from build123d import *

# Parameters (mm, degrees)
SKETCH_1_W            = 65
SKETCH_1_H            = 72
EXTRUDE_1_DEPTH       = 50
SKETCH_2_W            = 28
SKETCH_2_H            = 50
CUT_EXTRUDE_1_DEPTH   = 94.489304201
SKETCH_4_W            = 65
SKETCH_4_H            = 20
CUT_EXTRUDE_3_DEPTH   = 52
CHAMFER_1_SIZE        = 5
HOLE_WIZARD_9_0_9_1_D = 9
HOLE_WIZARD_8_0_8_1_D = 8
FILLET_1_R            = 1


with BuildPart() as part:
    # 草圖1 → 伸長1 (new, symmetric)
    with BuildSketch(Plane.XY):
        Rectangle(SKETCH_1_W, SKETCH_1_H)
    extrude(amount=EXTRUDE_1_DEPTH, both=True)

    # 草圖2 → 除料-伸長1 (cut, through all)
    with BuildSketch(Plane(origin=(0, 36, 0), x_dir=(1, 0, 0), z_dir=(0, 1, 0))):
        Rectangle(SKETCH_2_W, SKETCH_2_H)
    extrude(amount=-CUT_EXTRUDE_1_DEPTH, mode=Mode.SUBTRACT)

    # 草圖4 → 除料-伸長3 (cut)
    with BuildSketch(Plane(origin=(0, 36, 0), x_dir=(1, 0, 0), z_dir=(0, 1, 0))):
        with Locations((0, -40)):
            Rectangle(SKETCH_4_W, SKETCH_4_H)
        with Locations((0, 40)):
            Rectangle(SKETCH_4_W, SKETCH_4_H)
    extrude(amount=-CUT_EXTRUDE_3_DEPTH, mode=Mode.SUBTRACT)

    # 導角1
    chamfer_1_edges = [part.edges().sort_by_distance(p)[0] for p in [
        (32.5, -26, 50),
        (-32.5, -26, 50),
        (-32.5, -26, -50),
        (32.5, -26, -50),
    ]]
    chamfer(chamfer_1_edges, length=CHAMFER_1_SIZE)

    # Ø9.0 (9) 直徑孔1 (through all)
    with Locations(Plane(origin=(0, -16, 0), x_dir=(-1, 0, 0), z_dir=(0, 1, 0))):
        with Locations((25, -40), (-25, -40), (-25, 40), (25, 40)):
            Hole(HOLE_WIZARD_9_0_9_1_D / 2)

    # Ø8.0 (8) 直徑孔1 (through all)
    with Locations(Plane(origin=(0, -16, 0), x_dir=(-1, 0, 0), z_dir=(0, 1, 0))):
        with Locations((0, -40), (0, 40)):
            Hole(HOLE_WIZARD_8_0_8_1_D / 2)

    # 圓角1
    fillet_1_edges = [part.edges().sort_by_distance(p)[0] for p in [
        (-14, 0, 25),
        (-14, 0, -25),
        (14, 0, -25),
        (14, 0, 25),
    ]]
    fillet(fillet_1_edges, radius=FILLET_1_R)


solid = part.part
Could you check a few things on this model? Use its own coordinates, in mm. A direction names the side the tool comes from. Coordinates: 2 decimals unless noted, no trailing zeros. Order: outer loops, then holes, each group sorted by start corner. A loop starts at its lowest first (then second) coordinate and runs counter-clockwise, first axis right, second up. Notation, with made-up numbers: (52, 85.25) -> (80, 85.25) arc R20 ccw to (80, 92.25) -> close; hole circle Ø5 at (64, -24). An arc over 180 degrees is marked (long way). One line per item, written item: value. Start each with the question number.
1) I'm going to push flat-ended pins straight in: pin 1 (15.5 mm diameter, centred on x = -5, y = 8, fed in from -Z); pin 2 (7 mm diameter, centred on x = -25, z = -40, fed in from +Y); pin 3 (13 mm diameter, centred on x = 0, z = 40, fed in from +Y); pin 4 (13 mm diameter, centred on x = 4.5, y = 16, fed in from +Z). Where does each tip first touch, or does it pass through?
2) Imagine slicing it at A-A on x = 25. List the corners of the cut face in (y, z) for me.
3) If I drill on L1, parallel to Z at x = 0, y = -28.5; L2, parallel to Z at x = -25, y = -22.5; L3, parallel to X at y = -16, z = -10, over which ranges is the centre line in solid material (lowest first)? Write a range as [from, to].
4) Imagine slicing it at C-C on y = -28.5. List the corners of the cut face in (x, z) for me.
5) We'd pull the mould along X, two halves only. Please class faces 5 (the flat face through (32.5, -1, 1)), 6 (the flat face through (0, 1, -25)), 7 (the flat face through (-30, -26.1, 47.5)): +X half, -X half, draft (parallel to the pull), parting line (faces both ways), or undercut.
6) Which directions (+Z, -Z, +X, -X, +Y, -Y) give clear straight access to the entire face, cutting with the end or side of a thin tool? Please do faces 1 (the flat face through (0, 10, -30)), 2 (the flat face through (0, 1, 25)), 3 (the flat face through (-15, 36, 0)), 4 (the flat face through (0, 10, 30)).
7) Imagine slicing it at B-B on z = 40. List the corners of the cut face in (x, y) for me, plus the area to 3 significant figures.
8) Imagine slicing it at D-D on x = 0. List the corners of the cut face in (y, z) for me, plus the area to 3 significant figures.
Answer list:
1. pin 1: stops at z = -30
1. pin 2: passes through
1. pin 3: stops at y = -16
1. pin 4: stops at z = 30
2. outline: (-36, -50) -> (-16, -50) -> (-16, -44.5) -> (-36, -44.5) -> close; (-36, -35.5) -> (-16, -35.5) -> (-16, -30) -> (36, -30) -> (36, 30) -> (-16, 30) -> (-16, 35.5) -> (-36, 35.5) -> close; (-36, 44.5) -> (-16, 44.5) -> (-16, 50) -> (-36, 50) -> close
3. L1: z = [-50, -44], [-36, -25], [25, 36], [44, 50]
3. L2: z = [-50, -44.5], [-35.5, 35.5], [44.5, 50]
3. L3: x = [-32.5, -14], [14, 32.5]
4. outline: (-32.5, -45) -> (-27.5, -50) -> (27.5, -50) -> (32.5, -45) -> (32.5, 45) -> (27.5, 50) -> (-27.5, 50) -> (-32.5, 45) -> close; hole circle Ø9 at (-25, -40); hole circle Ø9 at (-25, 40); hole (-14, -24) arc R1 ccw to (-13, -25) -> (13, -25) arc R1 ccw to (14, -24) -> (14, 24) arc R1 ccw to (13, 25) -> (-13, 25) arc R1 ccw to (-14, 24) -> close; hole circle Ø8 at (0, -40); hole circle Ø8 at (0, 40); hole circle Ø9 at (25, -40); hole circle Ø9 at (25, 40)
5. face 5: +X half
5. face 6: undercut
5. face 7: -X half
6. face 1: -Z, +X, -X, +Y
6. face 2: +Y, -Y
6. face 3: +Z, -Z, +X, -X, +Y
6. face 4: +Z, +X, -X, +Y
7. outline: (-32.5, -36) -> (-29.5, -36) -> (-29.5, -16) -> (-32.5, -16) -> close; (-20.5, -36) -> (-4, -36) -> (-4, -16) -> (-20.5, -16) -> close; (4, -36) -> (20.5, -36) -> (20.5, -16) -> (4, -16) -> close; (29.5, -36) -> (32.5, -36) -> (32.5, -16) -> (29.5, -16) -> close
7. area: 780 mm2
8. outline: (-36, -50) -> (-16, -50) -> (-16, -44) -> (-36, -44) -> close; (-36, -36) -> (-16, -36) -> (-16, -30) -> (36, -30) -> (36, -25) -> (-36, -25) -> close; (-36, 25) -> (36, 25) -> (36, 30) -> (-16, 30) -> (-16, 36) -> (-36, 36) -> close; (-36, 44) -> (-16, 44) -> (-16, 50) -> (-36, 50) -> close
8. area: 1,200 mm2
